Geometry check sheet. Reference: the model listing, model coordinates, mm. A direction names the side the tool comes from. Coordinates: 2 decimals unless noted, no trailing zeros. Order: outer loops, then holes, each group sorted by start corner. A loop starts at its lowest first (then second) coordinate and runs counter-clockwise, first axis right, second up. Notation, with made-up numbers: (86, 50.25) -> (91, 50.25) arc R29 ccw to (91, 77.25) -> close; hole circle Ø1 at (6, 32.25). An arc over 180 degrees is marked (long way). Answer as CSV lines item,"result". Start each with the question number.
from build123d import *

# Parameters (mm, degrees)
SKETCH1_W           = 120
SKETCH1_H           = 120
SKETCH1_R           = 4.285714286
BOSS_EXTRUDE1_DEPTH = 10
SKETCH2_W           = 120
SKETCH2_H           = 120
SKETCH2_W_2         = 100
SKETCH2_H_2         = 100
BOSS_EXTRUDE2_DEPTH = 190
SKETCH3_R           = 3.25
CUT_EXTRUDE1_DEPTH  = 15
CUT_EXTRUDE2_REACH  = 122
SKETCH4_R           = 6.5


with BuildPart() as part:
    # Sketch1 → Boss-Extrude1 (new body)
    with BuildSketch(Plane(origin=(0, 0, 0), x_dir=(1, 0, 0), z_dir=(0, 1, 0))):
        Rectangle(SKETCH1_W, SKETCH1_H)
        Circle(SKETCH1_R, mode=Mode.SUBTRACT)
    extrude(amount=BOSS_EXTRUDE1_DEPTH)

    # Sketch2 → Boss-Extrude2 (add)
    with BuildSketch(Plane.XZ):
        Rectangle(SKETCH2_W, SKETCH2_H)
        Rectangle(SKETCH2_W_2, SKETCH2_H_2, mode=Mode.SUBTRACT)
    extrude(amount=BOSS_EXTRUDE2_DEPTH)

    # Sketch3 → Cut-Extrude1 (cut)
    with BuildSketch(Plane.XZ.offset(190)):
        with Locations((-55, -55)):
            Circle(SKETCH3_R)
        with Locations((55, 55)):
            Circle(SKETCH3_R)
        with Locations((-55, 55)):
            Circle(SKETCH3_R)
        with Locations((55, -55)):
            Circle(SKETCH3_R)
    extrude(amount=-CUT_EXTRUDE1_DEPTH, mode=Mode.SUBTRACT)

    # Sketch4 → Cut-Extrude2 (cut, up to next)
    with BuildSketch(Plane(origin=(0, 0, -60), x_dir=(-1, 0, 0), z_dir=(0, 0, -1)), mode=Mode.PRIVATE) as cut_extrude2_sk1:
        with Locations((0, -174.75)):
            Circle(SKETCH4_R)
    cut_extrude2_tool1 = extrude(cut_extrude2_sk1.sketch, amount=-CUT_EXTRUDE2_REACH, mode=Mode.PRIVATE) & part.part
    add(cut_extrude2_tool1.solids().sort_by_distance((0, -174.75, -60))[0], mode=Mode.SUBTRACT)


solid = part.part
Q1. Sectioned sample at A-A, the plane y = -75. Record the cut outline in (x, z), then the cut area to 3 significant figures.
Q2. Sectioned sample at C-C, the plane x = 14.5. Record the cut outline in (y, z).
Q3. Go/stop test with flat-tipped pins: pin 1 Ø1 at (x, z) = (31.5, -7.5) entering from -Y; pin 2 Ø11.5 at (x, y) = (0, -174.75) entering from -Z; pin 3 Ø10.5 at (x, z) = (55, 55) entering from -Y; pin 4 Ø2 at (x, z) = (54.5, 54) entering from -Y. Record where each tip stops, or that it passes through.
Q4. Sectioned sample at B-B, the plane z = -11. Record the cut outline in (x, y).
Q5. Access from +Z, -Z, +X, -X, +Y, -Y to the whole of each face (thin tool, end or side, straight path). Record for faces 1 (the flat face through (50, -94, -1)), 2 (the flat face through (0, -190, -53)).
Q6. Release check for a two-part mould opening along Z. For faces 3 (the flat face through (-50, -94, -1)), 4 (the cylindrical face through (1.409, -181.095, -55.07)), 5 (the flat face through (-1, -89, 60)), 6 (the flat face through (-1, -94, -50)) record: released by +Z, released by -Z, zero draft, split by the parting line, or undercut.
Q7. Thickness scan on L1, parallel to Z at x = -55, y = -184.25; L2, parallel to Z at x = -33, y = -48. Record the ranges inside material, lowest first.
Geometry results:
1,outline,"(-60, -60) -> (60, -60) -> (60, 60) -> (-60, 60) -> close; hole (-50, -50) -> (50, -50) -> (50, 50) -> (-50, 50) -> close"
1,area,"4,400 mm^2"
2,outline,"(-190, -60) -> (10, -60) -> (10, 60) -> (-190, 60) -> (-190, 50) -> (0, 50) -> (0, -50) -> (-190, -50) -> close"
3,pin 1,"stops at y = 0"
3,pin 2,"stops at z = 50"
3,pin 3,"stops at y = -190"
3,pin 4,"stops at y = -175"
4,outline,"(-60, -190) -> (-50, -190) -> (-50, 0) -> (50, 0) -> (50, -190) -> (60, -190) -> (60, 10) -> (-60, 10) -> close"
5,face 1,"-Y"
5,face 2,"+Z, -Z, +X, -X, -Y"
6,face 3,"undercut"
6,face 4,"zero draft"
6,face 5,"released by +Z"
6,face 6,"undercut"
7,L1,"z = -60 to -58.25, -51.75 to 51.75, 58.25 to 60"
7,L2,"z = -60 to -50, 50 to 60"
